```python
from build123d import *

# Parameters (mm, degrees)
BOSS_EXTRUDE1_DEPTH      = 15
BOSS_EXTRUDE1_DEPTH_BACK = 1
SKETCH1_W                = 30
SKETCH1_H                = 60
SKETCH2_R                = 3
CUT_EXTRUDE1_DEPTH       = 49
FILLET1_R                = 8
SKETCH6_W                = 30
SKETCH6_H                = 80
BOSS_EXTRUDE2_DEPTH      = 10
SKETCH7_R                = 3
CUT_EXTRUDE2_DEPTH       = 38
SKETCH8_R                = 3
CUT_EXTRUDE3_DEPTH       = 49
SKETCH11_W               = 10
SKETCH11_H               = 20
CUT_EXTRUDE4_DEPTH       = 30
FILLET2_R                = 15
FILLET3_R                = 25
CUT_EXTRUDE5_DEPTH       = 10
FILLET5_R                = 5


# Some blends are built 0.0001 mm under size
with BuildPart() as part:
    # Sketch1 → Boss-Extrude1 (new, two sides: drawn at the far end of the back side and taken through both)
    with BuildSketch(Plane.XY.offset(-BOSS_EXTRUDE1_DEPTH_BACK)):
        with Locations((15, -30)):
            Rectangle(SKETCH1_W, SKETCH1_H)
    extrude(amount=BOSS_EXTRUDE1_DEPTH + BOSS_EXTRUDE1_DEPTH_BACK)

    # Sketch2 → Cut-Extrude1 (cut)
    with BuildSketch(Plane.ZY):
        with Locations((7, -10)):
            Circle(SKETCH2_R)
    extrude(amount=-CUT_EXTRUDE1_DEPTH, mode=Mode.SUBTRACT)

    # Fillet1
    fillet1_edges = [part.edges().sort_by_distance(p)[0] for p in [
        (15, 0, 15),
        (15, 0, -1),
    ]]
    fillet(fillet1_edges, radius=FILLET1_R - 0.0001)  # a hair under: the kernel refuses the full size

    # Sketch6 → Boss-Extrude2 (add)
    with BuildSketch(Plane(origin=(0, -11.839573779, 32.528961614), x_dir=(1, 0, 0), z_dir=(0, 0.34202014332566943, -0.9396926207859081))):
        with Locations((15, 11.251255097)):
            Rectangle(SKETCH6_W, SKETCH6_H)
    extrude(amount=BOSS_EXTRUDE2_DEPTH)

    # Sketch7 → Cut-Extrude2 (cut)
    with BuildSketch(Plane(origin=(0, 0, -1), x_dir=(-1, 0, 0), z_dir=(0, 0, -1))):
        with Locations(Location((-15, -20, 0), (0, 0, 270))):
            Circle(SKETCH7_R)
        with Locations((-15, -30)):
            Circle(SKETCH7_R)
    extrude(amount=-CUT_EXTRUDE2_DEPTH, mode=Mode.SUBTRACT)

    # Sketch8 → Cut-Extrude3 (cut)
    with BuildSketch(Plane.ZY):
        with Locations((8, -50)):
            Circle(SKETCH8_R)
    extrude(amount=-CUT_EXTRUDE3_DEPTH, mode=Mode.SUBTRACT)

    # Sketch11 → Cut-Extrude4 (cut)
    with BuildSketch(Plane(origin=(0, 0, -1), x_dir=(-1, 0, 0), z_dir=(0, 0, -1))):
        with Locations((-15, -50)):
            Rectangle(SKETCH11_W, SKETCH11_H)
    extrude(amount=-CUT_EXTRUDE4_DEPTH, mode=Mode.SUBTRACT)

    # Fillet2
    fillet2_edges = [part.edges().sort_by_distance(p)[0] for p in [
        (25, -60, -1),
        (5, -60, -1),
    ]]
    fillet(fillet2_edges, radius=FILLET2_R)

    # Fillet3
    # the kernel refuses this fillet: 25 mm, written as the material it takes off along each edge
    with BuildSketch(Plane(origin=(0, -6.200849295, 101.092400265), x_dir=(1, 0, 0), z_dir=(0, 0.34202014332566943, -0.9396926207859082)), Plane(origin=(30, -6.200849295, 101.092400265), x_dir=(0, -0.9396926207859081, -0.3420201433256693), z_dir=(0, 0.34202014332566943, -0.9396926207859082))) as fillet3_piece_1:
        with BuildLine():
            CenterArc((FILLET3_R, FILLET3_R), FILLET3_R, 180, 90)
            Line((0, FILLET3_R), (0, 0))
            Line((0, 0), (FILLET3_R, 0))
        make_face()
    extrude(amount=135, mode=Mode.SUBTRACT)

    # Sketch12 → Cut-Extrude5 (cut)
    with BuildSketch(Plane(origin=(0, -8.419372346, 23.132035406), x_dir=(-1, 0, 0), z_dir=(0, 0.34202014332566943, -0.9396926207859082))):
        with BuildLine():
            Line((-15, 21.748370766), (-7.650260268, 21.748370766))
            ThreePointArc((-7.650260268, 21.748370766), (-15, 27.089106291), (-22.349739732, 21.748370766))
            Line((-22.349739732, 21.748370766), (-15, 21.748370766))
        make_face()
    extrude(amount=-CUT_EXTRUDE5_DEPTH, mode=Mode.SUBTRACT)

    # Fillet5
    fillet5_edges = [part.edges().sort_by_distance(p)[0] for p in [
        (15, 8.597209744, 39.967342501),
        (15, 12.017411178, 30.570416293),
    ]]
    fillet(fillet5_edges, radius=FILLET5_R - 0.0001)  # a hair under: the kernel refuses the full size


solid = part.part
```
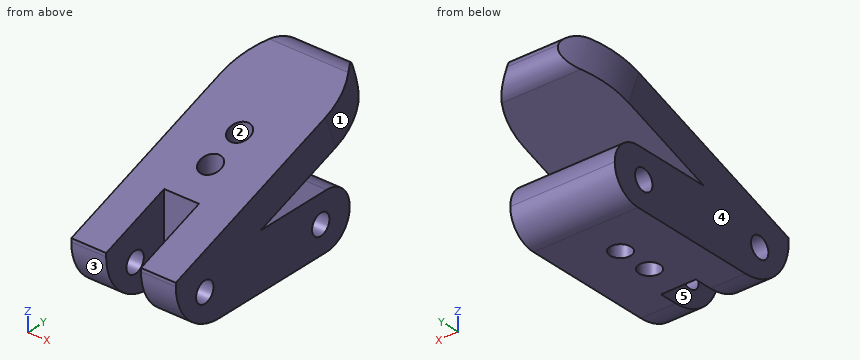
Here's how the part is built. I have some questions about the finished solid (model axes, mm). Face numbers are marked on the shaded views. A direction names the side the tool comes from. Round coordinates to 2 decimals unless told otherwise and drop trailing zeros. Order: outer loops, then holes, each group sorted by start corner. A loop starts at its lowest first (then second) coordinate and runs counter-clockwise, first axis right, second up. Notation, with made-up numbers: M 85.5,45.5 L 96.5,45.5 A18 ccw 96.5,51.5 Z; hole C 80.5,56.5 d6. An arc over 180 degrees is marked long. Answer in a Markdown table with one row per item.
Item 1: Thinking about a two-plate mould opening in Y: for the marked faces 1, 2 and 3, which applies, +Y half, -Y half, draft (parallel to the pull), parting line (faces both ways), or undercut?
A:
| item | result |
|---|---|
| face 1 | +Y half |
| face 2 | undercut |
| face 3 | -Y half |
Item 2: If I drill on L1, parallel to Y at x = 15, z = 7; L2, parallel to X at y = -45.5, z = 1; L3, parallel to Y at x = 2, z = 8, over which ranges is the centre line in solid material (lowest first)? Write a range as from..to.
A:
| item | result |
|---|---|
| L1 | y = -40..-33, -27..-23, -17..-13, -7..0 |
| L2 | x = 0..10, 20..30 |
| L3 | y = -58.75..-53, -47..-12.83, -7.17..-0.06 |
Item 3: I'm going to push flat-ended pins straight in: pin 1 (3.5 mm diameter, centred on y = -50, z = 8, fed in from +X); pin 2 (12 mm diameter, centred on x = 13, y = -45, fed in from +Z); pin 3 (4 mm diameter, centred on x = 18.5, y = -50, fed in from +Z); pin 4 (8 mm diameter, centred on x = 17.5, z = 14, fed in from +Y). Where does each tip first touch, or does it pass through?
A:
| item | result |
|---|---|
| pin 1 | passes through |
| pin 2 | stops at z = 22.64 |
| pin 3 | stops at z = 19.12 |
| pin 4 | stops at y = -0.58 |
Item 4: Imagine slicing it at D-D, the plane z = 21. Write out the boundary of the cut face in (x, y), and give its area (3 significant figures).
A:
| item | result |
|---|---|
| outline | M 0,-43.52 L 10,-43.52 L 10,-40 L 20,-40 L 20,-43.52 L 30,-43.52 L 30,-14.28 L 0,-14.28 Z; hole C 15,-30 d6; hole C 15,-20 d6 |
| area | 785 mm2 |
Item 5: Imagine slicing it at B-B, the plane z = 8. Write out the boundary of the cut face in (x, y), and give its area (3 significant figures).
A:
| item | result |
|---|---|
| outline | M 0,-58.75 L 10,-58.75 L 10,-53 L 0,-53 Z; M 0,-47 L 10,-47 L 10,-40 L 20,-40 L 20,-47 L 30,-47 L 30,-12.83 L 0,-12.83 Z; M 0,-7.17 L 30,-7.17 L 30,-0.06 L 0,-0.06 Z; M 20,-58.75 L 30,-58.75 L 30,-53 L 20,-53 Z; hole C 15,-30 d6; hole C 15,-20 d6 |
| area | 1,230 mm2 |
Item 6: Imagine slicing it at A-A, the plane x = 14. State how many separate pieces and enclosed holes the cut face has, and give its area (3 significant figures).
A:
| item | result |
|---|---|
| separate pieces | 5 |
| enclosed holes | 1 |
| area | 793 mm2 |
Item 7: For the marked faces 4 and 5, which set-ups out of +Z, -Z, +X, -X, +Y, -Y let a thin tool reach every point of the face, with its end or its side?
A:
| item | result |
|---|---|
| face 4 | +Z, -Z, -X, +Y, -Y |
| face 5 | +Z, -Z, -Y |
Item 8: Imagine slicing it at C-C, the plane y = -50. Write out the boundary of the cut face in (x, z).
A:
| item | result |
|---|---|
| outline | M 0,-0.14 L 10,-0.14 L 10,5 L 0,5 Z; M 0,11 L 10,11 L 10,18.64 L 0,18.64 Z; M 20,-0.14 L 30,-0.14 L 30,5 L 20,5 Z; M 20,11 L 30,11 L 30,18.64 L 20,18.64 Z |
